```python
from build123d import *

# Parameters (mm, degrees)
BOSS_EXTRUDE1_DEPTH = 1
SKETCH2_R           = 7.5
BOSS_EXTRUDE2_DEPTH = 0.1
DOME1_FACE_RADIUS   = 7.5
DOME1_HEIGHT        = 8
SKETCH3_R           = 1.75
CUT_EXTRUDE1_DEPTH  = 68.203209981
SKETCH5_R           = 2.75
CUT_EXTRUDE2_DEPTH  = 7.1
SKETCH6_W           = 0.5
SKETCH6_H           = 38.067336288
BOSS_EXTRUDE3_DEPTH = 0.1
BOSS_EXTRUDE6_DEPTH = 0.1


with BuildPart() as part:
    # Sketch1 → Boss-Extrude1 (new body)
    with BuildSketch(Plane(origin=(0, 0, 0), x_dir=(1, 0, 0), z_dir=(0, 1, 0))):
        with BuildLine():
            Line((-5, 45), (-5, 5.590169944))
            ThreePointArc((-5, 5.590169944), (-6.495190528, 3.75), (-7.341229183, 1.535042047))
            Line((-7.341229183, 1.535042047), (-41.47114317, -18.169872981))
            ThreePointArc((-41.47114317, -18.169872981), (-43.301270189, -25), (-36.47114317, -26.830127019))
            Line((-36.47114317, -26.830127019), (-2.341229183, -7.125211991))
            ThreePointArc((-2.341229183, -7.125211991), (0, -7.5), (2.341229183, -7.125211991))
            Line((2.341229183, -7.125211991), (36.47114317, -26.830127019))
            ThreePointArc((36.47114317, -26.830127019), (43.301270189, -25), (41.47114317, -18.169872981))
            Line((41.47114317, -18.169872981), (7.341229183, 1.535042047))
            ThreePointArc((7.341229183, 1.535042047), (6.495190528, 3.75), (5, 5.590169944))
            Line((5, 5.590169944), (5, 45))
            ThreePointArc((5, 45), (0, 50), (-5, 45))
        make_face()
    extrude(amount=BOSS_EXTRUDE1_DEPTH)

    # Sketch2 → Boss-Extrude2 (add)
    with BuildSketch(Plane(origin=(0, 1, 0), x_dir=(1, 0, 0), z_dir=(0, 1, 0))):
        with Locations(Location((0, 0, 0), (0, 0, 48.189685104))):
            Circle(SKETCH2_R)
    extrude(amount=BOSS_EXTRUDE2_DEPTH)

    # Dome1: a dome of height H over a round flat face of radius A is a cap of a sphere of radius (A * A + H * H) / (2 * H)
    dome1_r = (DOME1_FACE_RADIUS * DOME1_FACE_RADIUS + DOME1_HEIGHT * DOME1_HEIGHT) / (2 * DOME1_HEIGHT)
    dome1_base = Plane((0, 1.1, 0), z_dir=(0, 1, 0))
    with Locations(dome1_base.offset(DOME1_HEIGHT - dome1_r)):
        dome1_ball = Sphere(dome1_r, mode=Mode.PRIVATE)
    add(split(dome1_ball, bisect_by=dome1_base, keep=Keep.TOP, mode=Mode.PRIVATE))

    # Sketch3 → Cut-Extrude1 (cut, through all)
    with BuildSketch(Plane.XZ):
        with Locations(Location((0, 0, 0), (0, 0, 270))):
            Circle(SKETCH3_R)
    extrude(amount=-CUT_EXTRUDE1_DEPTH, mode=Mode.SUBTRACT)

    # Sketch5 → Cut-Extrude2 (cut)
    with BuildSketch(Plane.XZ):
        with Locations(Location((0, 0, 0), (0, 0, 270))):
            Circle(SKETCH5_R)
    extrude(amount=-CUT_EXTRUDE2_DEPTH, mode=Mode.SUBTRACT)

    # Sketch6 → Boss-Extrude3 (add)
    with BuildSketch(Plane(origin=(0, 1, 0), x_dir=(1, 0, 0), z_dir=(0, 1, 0))):
        with Locations((-1, 25.721859363)):
            Rectangle(SKETCH6_W, SKETCH6_H)
        with Locations((0, 25.721859363)):
            Rectangle(SKETCH6_W, SKETCH6_H)
        with Locations((1, 25.721859363)):
            Rectangle(SKETCH6_W, SKETCH6_H)
        Polygon((39.384423781, -21.295231999), (6.417143501, -2.261563855), (6.167143501, -2.694576557), (39.134423781, -21.728244701), align=None)
        Polygon((38.884423781, -22.161257403), (5.917143501, -3.127589259), (5.667143501, -3.560601961), (38.634423781, -22.594270105), align=None)
        Polygon((38.384423781, -23.027282807), (5.417143501, -3.993614663), (5.167143501, -4.426627364), (38.134423781, -23.460295508), align=None)
        Polygon((-38.134423781, -23.460295508), (-5.167143501, -4.426627364), (-5.417143501, -3.993614663), (-38.384423781, -23.027282807), align=None)
        Polygon((-38.634423781, -22.594270105), (-5.667143501, -3.560601961), (-5.917143501, -3.127589259), (-38.884423781, -22.161257403), align=None)
        Polygon((-39.134423781, -21.728244701), (-6.167143501, -2.694576557), (-6.417143501, -2.261563855), (-39.384423781, -21.295231999), align=None)
    extrude(amount=BOSS_EXTRUDE3_DEPTH)

    # Sketch11 → Boss-Extrude6 (add)
    with BuildSketch(Plane.XZ):
        with BuildLine():
            Line((17.740956204, 16.443798031), (-17.759043796, 16.443798031))
            Line((-17.759043796, 16.443798031), (-17.759043796, -12.556201969))
            ThreePointArc((-17.759043796, -12.556201969), (-15.097202282, -18.94586135), (-8.686211126, -21.555907264))
            Line((-8.686211126, -21.555907264), (8.813788874, -21.555907264))
            ThreePointArc((8.813788874, -21.555907264), (15.130615586, -18.894360454), (17.740956204, -12.556201969))
            Line((17.740956204, -12.556201969), (17.740956204, 16.443798031))
        make_face()
    extrude(amount=BOSS_EXTRUDE6_DEPTH)


solid = part.part
```
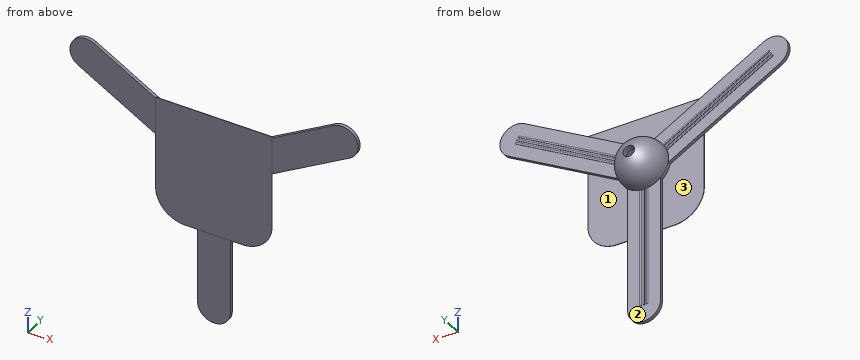
Design review of the part built by this model. Coordinates are the model's own, in mm. Face numbers are marked on the shaded views. A direction names the side the tool comes from. Give positions to 0.01 mm unless a question says otherwise; leave off trailing zeros. Order: outer loops, then holes, each group sorted by start corner. A loop starts at its lowest first (then second) coordinate and runs counter-clockwise, first axis right, second up. Notation, with made-up numbers: (19, -2) -> (56, -2) arc R17 ccw to (56, 5) -> close; hole circle Ø10 at (59, 86). An arc over 180 degrees is marked (long way). Write each question's results on one line, items separated by ' | '. Start each with the question number.
Q1. Wall thickness on L1, parallel to Y at x = -18, z = 14; L2, parallel to X at y = 4.75, z = 0; L3, parallel to Z at x = -2.5, y = 3.5: over which ranges is each line inside the solid? List them lowest first. Write a range as from..to.
Q2. Add section A-A on z = -27.5. Give the boundary of the cut face in (x, y), and give its area (4 significant figures).
Q3. Add section D-D on z = -11.5. Give the boundary of the cut face in (x, y), and give its area (3 significant figures).
Q4. Machinability: for the marked faces 1, 2 and 3, which of the approach directions +Z, -Z, +X, -X, +Y, -Y give a long, thin tool a straight path to every point of the face, cutting with its end or side? Answer none if there is none.
Q5. Add section C-C on y = 3. Give the boundary of the cut face in (x, z), and give its area (3 significant figures).
Q6. For pin 1 (14 mm diameter, centred on x = -11, z = -7.5, fed in from +Y); pin 2 (15.5 mm diameter, centred on x = 28.5, z = 12, fed in from +Y); pin 3 (1.5 mm diameter, centred on x = -6, y = 5.5, fed in from -Z), all flat-tipped, find the tip position at first contact; note any pin that passes through.
Q7. Add section B-B on x = 15. Give the boundary of the cut face in (y, z).
Found:
1) L1: y = 0..1 | L2: x = -6.82..-2.75, 2.75..6.82 | L3: z = -6.82..-1.15, 1.15..6.82
2) outline: (-5, 0) -> (5, 0) -> (5, 1) -> (1.25, 1) -> (1.25, 1.1) -> (0.75, 1.1) -> (0.75, 1) -> (0.25, 1) -> (0.25, 1.1) -> (-0.25, 1.1) -> (-0.25, 1) -> (-0.75, 1) -> (-0.75, 1.1) -> (-1.25, 1.1) -> (-1.25, 1) -> (-5, 1) -> close | area: 10.15 mm2
3) outline: (-17.76, -0.1) -> (17.74, -0.1) -> (17.74, 0) -> (5, 0) -> (5, 1) -> (1.25, 1) -> (1.25, 1.1) -> (0.75, 1.1) -> (0.75, 1) -> (0.25, 1) -> (0.25, 1.1) -> (-0.25, 1.1) -> (-0.25, 1) -> (-0.75, 1) -> (-0.75, 1.1) -> (-1.25, 1.1) -> (-1.25, 1) -> (-5, 1) -> (-5, 0) -> (-17.76, 0) -> close | area: 13.7 mm2
4) face 1: -Z, +X, +Y | face 2: -Z, +Y | face 3: -Z, -X, +Y
5) outline: circle Ø14.76 at (0, 0); hole circle Ø5.5 at (0, 0) | area: 147 mm2
6) pin 1: stops at y = 5.66 | pin 2: stops at y = 1.1 | pin 3: stops at z = -3.92
7) outline: (-0.1, -19.02) -> (0, -19.02) -> (0, 2.89) -> (1, 2.89) -> (1, 7.22) -> (1.1, 7.22) -> (1.1, 7.79) -> (1, 7.79) -> (1, 8.37) -> (1.1, 8.37) -> (1.1, 8.95) -> (1, 8.95) -> (1, 9.53) -> (1.1, 9.53) -> (1.1, 10.1) -> (1, 10.1) -> (1, 14.43) -> (0, 14.43) -> (0, 16.44) -> (-0.1, 16.44) -> close
